Autodesk Inventor part; units mm, degrees
ref_plane "YZ Plane" through (0, 0, 0) normal (1, 0, 0) x (0, 1, 0)
ref_plane "XZ Plane" through (0, 0, 0) normal (0, 1, 0) x (-1, 0, 0)
ref_plane "XY Plane" through (0, 0, 0) normal (0, 0, 1) x (1, 0, 0)
sketch "Sketch1" plane through (0, 0, 0) normal (0, 1, 0) x (-1, 0, 0)
  circle A0 centre (-336.55, 0) radius 3.3782
  circle A1 centre (-234.3065, 241.5985) radius 3.3782
  circle A2 centre (-241.5985, 234.3065) radius 3.3782
  circle A3 centre (87.8158, 336.55) radius 3.3782
  circle A4 centre (0, 336.55) radius 3.3782
  arc A5 (0, 342.9) -> (-342.9, 0) centre (0, 0) ccw
  arc A6 (0, 330.2) -> (-330.2, 0) centre (0, 0) ccw
  line L0 (-342.9, 0) -> (-342.9, -101.6)
  line L1 (-342.9, -101.6) -> (-330.2, -101.6)
  line L2 (-330.2, -101.6) -> (-330.2, 0)
  circle A7 centre (-336.55, -9.525) radius 3.3782
  circle A8 centre (-336.55, -19.05) radius 3.3782
  circle A9 centre (-336.55, -28.575) radius 3.3782
  circle A10 centre (-336.55, -38.1) radius 3.3782
  circle A11 centre (-336.55, -47.625) radius 3.3782
  circle A12 centre (-336.55, -57.15) radius 3.3782
  circle A13 centre (-336.55, -66.675) radius 3.3782
  circle A14 centre (-336.55, -76.2) radius 3.3782
  circle A15 centre (-336.55, -85.725) radius 3.3782
  circle A16 centre (-336.55, -95.25) radius 3.3782
  line L3 (0, 330.2) -> (101.6, 330.2)
  line L4 (101.6, 330.2) -> (101.6, 342.9)
  line L5 (101.6, 342.9) -> (0, 342.9)
  circle A17 centre (-10.3511, 336.3908) radius 3.3782
  circle A18 centre (-20.6925, 335.9133) radius 3.3782
  circle A19 centre (-31.0142, 335.1179) radius 3.3782
  circle A20 centre (-41.3066, 334.0055) radius 3.3782
  circle A21 centre (-51.5599, 332.577) radius 3.3782
  circle A22 centre (-61.7645, 330.8339) radius 3.3782
  circle A23 centre (-71.9106, 328.7777) radius 3.3782
  circle A24 centre (-81.9886, 326.4104) radius 3.3782
  circle A25 centre (-91.9891, 323.7343) radius 3.3782
  circle A26 centre (-101.9026, 320.7519) radius 3.3782
  circle A27 centre (-111.7196, 317.466) radius 3.3782
  circle A28 centre (-121.4309, 313.8797) radius 3.3782
  circle A29 centre (-131.0273, 309.9964) radius 3.3782
  circle A30 centre (-140.4997, 305.8198) radius 3.3782
  circle A31 centre (-149.8392, 301.3538) radius 3.3782
  circle A32 centre (-159.037, 296.6027) radius 3.3782
  circle A33 centre (-168.0842, 291.5709) radius 3.3782
  circle A34 centre (-176.9724, 286.2633) radius 3.3782
  circle A35 centre (-185.6932, 280.6848) radius 3.3782
  circle A36 centre (-194.2382, 274.8407) radius 3.3782
  circle A37 centre (-202.5995, 268.7366) radius 3.3782
  circle A38 centre (-210.769, 262.3782) radius 3.3782
  circle A39 centre (-218.7392, 255.7715) radius 3.3782
  circle A40 centre (-226.5024, 248.9228) radius 3.3782
  circle A41 centre (-336.3908, 10.3511) radius 3.3782
  circle A42 centre (-335.9133, 20.6925) radius 3.3782
  circle A43 centre (-335.1179, 31.0142) radius 3.3782
  circle A44 centre (-334.0055, 41.3066) radius 3.3782
  circle A45 centre (-332.577, 51.5599) radius 3.3782
  circle A46 centre (-330.8339, 61.7645) radius 3.3782
  circle A47 centre (-328.7777, 71.9106) radius 3.3782
  circle A48 centre (-326.4104, 81.9886) radius 3.3782
  circle A49 centre (-323.7343, 91.9891) radius 3.3782
  circle A50 centre (-320.7519, 101.9026) radius 3.3782
  circle A51 centre (-317.466, 111.7196) radius 3.3782
  circle A52 centre (-313.8797, 121.4309) radius 3.3782
  circle A53 centre (-309.9964, 131.0273) radius 3.3782
  circle A54 centre (-305.8198, 140.4997) radius 3.3782
  circle A55 centre (-301.3538, 149.8392) radius 3.3782
  circle A56 centre (-296.6027, 159.037) radius 3.3782
  circle A57 centre (-291.5709, 168.0842) radius 3.3782
  circle A58 centre (-286.2633, 176.9724) radius 3.3782
  circle A59 centre (-280.6848, 185.6932) radius 3.3782
  circle A60 centre (-274.8407, 194.2382) radius 3.3782
  circle A61 centre (-268.7366, 202.5995) radius 3.3782
  circle A62 centre (-262.3782, 210.769) radius 3.3782
  circle A63 centre (-255.7715, 218.7392) radius 3.3782
  circle A64 centre (-248.9228, 226.5024) radius 3.3782
  circle A65 centre (9.525, 336.55) radius 3.3782
  circle A66 centre (19.05, 336.55) radius 3.3782
  circle A67 centre (28.575, 336.55) radius 3.3782
  circle A68 centre (38.1, 336.55) radius 3.3782
  circle A69 centre (47.625, 336.55) radius 3.3782
  circle A70 centre (57.15, 336.55) radius 3.3782
  circle A71 centre (66.675, 336.55) radius 3.3782
  circle A72 centre (76.2, 336.55) radius 3.3782
  line L6 (0, 325.5916) -> (0, 330.2)
  line L7 (0, 342.9) -> (0, 348.9307)
  dimension "d2" = 101.6
  dimension "d5" = 9.525
  dimension "d10" = 101.6
  dimension "d13" = 42.3
  dimension "d17" = 42.3
  dimension "d21" = 9.525
extrude "Extrusion1" add sketch "Sketch1" along normal blind 63.5
properties part number "Runner Rails 6 v1" material "Polycarbonate, Clear"
Verification items for the finished model (mm, model axes). A direction names the side the tool comes from. Coordinates: 2 decimals unless noted, no trailing zeros. Put each result on its own line as item: value. Start each with the question number.
1. Cross-section at A-A, the plane y = 52.5. Count the separate pieces of the cut face and the enclosed holes in it, then the cut area to 3 significant figures.
2. Material ranges on L1, parallel to X at y = 47, z = 303.5; L2, parallel to X at y = 6, z = 156; L3, parallel to Z at x = 263.5, y = 3.5, recorded low to high. Write a range as [from, to].
3. Access from +Z, -Z, +X, -X, +Y, -Y to the whole of each face (thin tool, end or side, straight path). Record for faces 1 (the cylindrical face through (245.118, 31.306, 239.786)), 2 (the flat face through (-50, 31, 330.2)).
4. Go/stop test with flat-tipped pins: pin 1 Ø4 at (x, z) = (336.55, 0) entering from -Y; pin 2 Ø10 at (x, y) = (223, 19.5) entering from +Z; pin 3 Ø1 at (y, z) = (43.5, -41) entering from -X; pin 4 Ø5 at (x, y) = (238, 30) entering from +Z. Record where each tip stops, or that it passes through.
Computed:
1. separate pieces: 1
1. enclosed holes: 71
1. area: 6,750 mm2
2. L1: [130.08, 138.04], [142.96, 147.23], [152.45, 159.59]
2. L2: [291.03, 295.12], [298.08, 305.36]
2. L3: [199, 207.58], [213.96, 219.43]
3. face 1: +Z, +X, +Y, -Y
3. face 2: -Z, -X, +Y, -Y
4. pin 1: through
4. pin 2: z = 264.68
4. pin 3: x = 330.2
4. pin 4: z = 249.24
